Read the model definition and answer for the solid it produces. Units are mm, in the model's axes. A direction names the side the tool comes from. Round coordinates to 2 decimals unless told otherwise and drop trailing zeros. Order: outer loops, then holes, each group sorted by start corner. A loop starts at its lowest first (then second) coordinate and runs counter-clockwise, first axis right, second up. Notation, with made-up numbers: (36, 78) -> (78, 78) arc R25 ccw to (78, 102) -> close; hole circle Ø10 at (70.25, 89.25). An arc over 180 degrees is marked (long way). Answer as a JSON object with one key per item and string values. Group by question number.
Item 1: The mould has two halves that part along X. Classify faces 1 (the flat face through (58.214, 0.986, 75.762)), 2 (the cylindrical face through (34.012, 0.986, 148.907)), 3 (the cylindrical face through (50.323, 0.986, 128.817)), 4 (the flat face through (-13.159, 0.986, 177.135)): pulls with the +X half, pulls with the -X half, needs draft (parallel to the pull), parting line crosses it, or undercut.
Item 2: For faces 5 (the flat face through (24.341, 0.986, 167.135)), 6 (the cylindrical face through (-16.806, 0.986, -22.588)), 7 (the flat face through (85, 1, 62.9)), determine the directions among +Z, -Z, +X, -X, +Y, -Y from which every point of the face is accessible in a straight line to the end or side of a thin tool.
Item 3: Section A-A, the plane x = 46 is taken. Write down the section's boundary in (y, z).
Item 4: Consider probe 1 along Z at (x, y) = (71, 0.25); probe 2 along Z at (x, y) = (42.5, 1.85); probe 3 along X at (y, z) = (0.1, -4.5). Determine where each line is inside the solid, lowest interval first. Write a range as from..to.
Item 5: Section C-C, the plane z = 166 is taken. Write down the section's boundary in (x, y), plus the area to 3 significant figures.
Item 6: Section B-B, the plane y = 1.3 is taken. Count the separate pieces of the cut face and the enclosed holes in it, plus the area to 3 significant figures.
from build123d import *

# Parameters (mm, degrees)
BASE_DEPTH               = 2
ESBO_O2_R                = 1
FURO_BRACKET_MOTOR_DEPTH = 3
ESBO_O4_W                = 60
ESBO_O4_H                = 70
ENCAIXE_PCB_DEPTH        = 236.289901939
ESBO_O6_R                = 1.5
PARAFUSO_PCB_DEPTH       = 236.289901939
ESBO_O7_R                = 2
ENFORCA_GATO_DEPTH       = 236.289901939
ESBO_O8_R                = 1.5
PARAFUSO_APOIO_DEPTH     = 10
ESBO_O9_R                = 1
ESBO_O9_R_2              = 1.6
ESBO_O9_W                = 63.64
ESBO_O9_H                = 16
ESBO_O9_W_2              = 8.7
ESBO_O9_H_2              = 4
CORTE_EXTRUS_O1_DEPTH    = 10


with BuildPart() as part:
    # Esboço1 → Base (new body)
    with BuildSketch(Plane(origin=(0, 0, 0), x_dir=(1, 0, 0), z_dir=(0, 1, 0))):
        with BuildLine():
            Line((-18.088885989, 17.941465294), (-18.088885989, 19.441465294))
            ThreePointArc((-18.088885989, 19.441465294), (-16.770866504, 22.623445809), (-13.588885989, 23.941465294))
            Line((-13.588885989, 23.941465294), (97.411114011, 23.941465294))
            ThreePointArc((97.411114011, 23.941465294), (100.593094526, 22.623445809), (101.911114011, 19.441465294))
            Line((101.911114011, 19.441465294), (101.911114011, 17.941465294))
            Line((101.911114011, 17.941465294), (101.911114011, -45.8528642))
            ThreePointArc((101.911114011, -45.8528642), (100.781222343, -50.470350333), (97.646878374, -54.044384643))
            Line((97.646878374, -54.044384643), (71.911114011, -72.064760852))
            Line((71.911114011, -72.064760852), (61.911114011, -72.064760852))
            Line((61.911114011, -72.064760852), (54.411114011, -79.564760852))
            Line((54.411114011, -79.564760852), (54.411114011, -162.064760852))
            Line((54.411114011, -162.064760852), (64.411114011, -172.064760852))
            Line((64.411114011, -172.064760852), (91.911114011, -172.064760852))
            Line((91.911114011, -172.064760852), (101.911114011, -182.064760852))
            Line((101.911114011, -182.064760852), (101.911114011, -202.064760852))
            Line((101.911114011, -202.064760852), (91.911114011, -212.064760852))
            Line((91.911114011, -212.064760852), (-8.088885989, -212.064760852))
            Line((-8.088885989, -212.064760852), (-18.088885989, -202.064760852))
            Line((-18.088885989, -202.064760852), (-18.088885989, -182.064760852))
            Line((-18.088885989, -182.064760852), (-8.088885989, -172.064760852))
            Line((-8.088885989, -172.064760852), (19.411114011, -172.064760852))
            Line((19.411114011, -172.064760852), (29.411114011, -162.064760852))
            Line((29.411114011, -162.064760852), (29.411114011, -79.564760852))
            Line((29.411114011, -79.564760852), (21.911114011, -72.064760852))
            Line((21.911114011, -72.064760852), (11.911114011, -72.064760852))
            Line((11.911114011, -72.064760852), (-13.824650353, -54.044384643))
            ThreePointArc((-13.824650353, -54.044384643), (-16.958994321, -50.470350333), (-18.088885989, -45.8528642))
            Line((-18.088885989, -45.8528642), (-18.088885989, 17.941465294))
        make_face()
    extrude(amount=BASE_DEPTH)

    # Esboço2 → Furo Bracket Motor (cut)
    with BuildSketch(Plane(origin=(0, 2, 0), x_dir=(1, 0, 0), z_dir=(0, 1, 0))):
        with Locations(Location((-13.588885989, 19.021465294, 0), (0, 0, 270))):
            Circle(ESBO_O2_R)
        with Locations(Location((-13.588885989, 1.021465294, 0), (0, 0, 270))):
            Circle(ESBO_O2_R)
        with Locations(Location((97.411114011, 1.021465294, 0), (0, 0, 90))):
            Circle(ESBO_O2_R)
        with Locations(Location((97.411114011, 19.021465294, 0), (0, 0, 90))):
            Circle(ESBO_O2_R)
    extrude(amount=-FURO_BRACKET_MOTOR_DEPTH, mode=Mode.SUBTRACT)

    # Esboço4 → Encaixe PCB (cut, through all)
    with BuildSketch(Plane.XZ):
        with Locations((41.911114011, 24.063534706)):
            Rectangle(ESBO_O4_W, ESBO_O4_H)
    extrude(amount=-ENCAIXE_PCB_DEPTH, mode=Mode.SUBTRACT)

    # Esboço6 → Parafuso PCB (cut, through all)
    with BuildSketch(Plane.XZ):
        with Locations(Location((16.911114011, 64.063534706, 0), (0, 0, 270))):
            Circle(ESBO_O6_R)
        with Locations(Location((66.911114011, 64.063534706, 0), (0, 0, 270))):
            Circle(ESBO_O6_R)
        with Locations(Location((66.911114011, -15.936465294, 0), (0, 0, 270))):
            Circle(ESBO_O6_R)
        with Locations(Location((16.911114011, -15.936465294, 0), (0, 0, 270))):
            Circle(ESBO_O6_R)
    extrude(amount=-PARAFUSO_PCB_DEPTH, mode=Mode.SUBTRACT)

    # Esboço7 → Enforca Gato (cut, through all)
    with BuildSketch(Plane.XZ):
        with Locations(Location((33.411114011, 90.814760852, 0), (0, 0, 270))):
            Circle(ESBO_O7_R)
        with Locations(Location((33.411114011, 110.814760852, 0), (0, 0, 270))):
            Circle(ESBO_O7_R)
        with Locations(Location((33.411114011, 130.814760852, 0), (0, 0, 270))):
            Circle(ESBO_O7_R)
        with Locations(Location((33.411114011, 150.814760852, 0), (0, 0, 270))):
            Circle(ESBO_O7_R)
        with Locations(Location((50.411114011, 150.814760852, 0), (0, 0, 90))):
            Circle(ESBO_O7_R)
        with Locations(Location((50.411114011, 130.814760852, 0), (0, 0, 90))):
            Circle(ESBO_O7_R)
        with Locations(Location((50.411114011, 110.814760852, 0), (0, 0, 90))):
            Circle(ESBO_O7_R)
        with Locations(Location((50.411114011, 90.814760852, 0), (0, 0, 90))):
            Circle(ESBO_O7_R)
    extrude(amount=-ENFORCA_GATO_DEPTH, mode=Mode.SUBTRACT)

    # Esboço8 → Parafuso Apoio (cut)
    with BuildSketch(Plane.XZ):
        with Locations(Location((95.911114011, 182.064760852, 0), (0, 0, 270))):
            Circle(ESBO_O8_R)
        with Locations(Location((95.911114011, 202.064760852, 0), (0, 0, 270))):
            Circle(ESBO_O8_R)
        with Locations(Location((-12.088885989, 202.064760852, 0), (0, 0, 270))):
            Circle(ESBO_O8_R)
        with Locations(Location((-12.088885989, 182.064760852, 0), (0, 0, 270))):
            Circle(ESBO_O8_R)
    extrude(amount=-PARAFUSO_APOIO_DEPTH, mode=Mode.SUBTRACT)

    # Esboço9 → Corte-extrusão1 (cut)
    with BuildSketch(Plane(origin=(0, 2, 0), x_dir=(1, 0, 0), z_dir=(0, 1, 0))):
        with Locations(Location((76.731114011, -197.064760852, 0), (0, 0, 270))):
            Circle(ESBO_O9_R)
        with Locations(Location((7.091114011, -197.064760852, 0), (0, 0, 270))):
            Circle(ESBO_O9_R)
        with Locations(Location((-0.438885989, -202.924760852, 0), (0, 0, 270))):
            Circle(ESBO_O9_R_2)
        with Locations(Location((84.261114011, -202.924760852, 0), (0, 0, 90))):
            Circle(ESBO_O9_R_2)
        with Locations((41.911114011, -197.064760852)):
            Rectangle(ESBO_O9_W, ESBO_O9_H)
        with Locations((-0.438885989, -193.064760852)):
            Rectangle(ESBO_O9_W_2, ESBO_O9_H_2)
        with Locations((84.261114011, -193.064760852)):
            Rectangle(ESBO_O9_W_2, ESBO_O9_H_2)
    extrude(amount=-CORTE_EXTRUS_O1_DEPTH, mode=Mode.SUBTRACT)


solid = part.part
Values found:
{
 "1": {"face 1": "pulls with the +X half", "face 2": "undercut", "face 3": "undercut", "face 4": "pulls with the -X half"},
 "2": {"face 5": "-X, +Y, -Y", "face 6": "-Z, -X, +Y, -Y", "face 7": "+X, +Y, -Y"},
 "3": {"outline": "(0, -23.94) -> (2, -23.94) -> (2, -10.94) -> (0, -10.94) -> close; (0, 59.06) -> (2, 59.06) -> (2, 189.06) -> (0, 189.06) -> close; (0, 205.06) -> (2, 205.06) -> (2, 212.06) -> (0, 212.06) -> close"},
 "4": {"probe 1": "-23.94..-10.94, 59.06..72.06, 172.06..189.06, 205.06..212.06", "probe 2": "-23.94..-10.94, 59.06..189.06, 205.06..212.06", "probe 3": "-18.09..11.91, 71.91..101.91"},
 "5": {"outline": "(25.48, 0) -> (58.35, 0) -> (58.35, 2) -> (25.48, 2) -> close", "area": "65.7 mm2"},
 "6": {"separate pieces": "1", "enclosed holes": "28", "area": "12,700 mm2"}
}
